Here's how the part is built. I have some questions about the finished solid (model axes, mm). A direction names the side the tool comes from. Give positions to 0.01 mm unless a question says otherwise; leave off trailing zeros. Write each loop counter-clockwise with the first axis right and the second up, starting at its lowest first coordinate (ties: lowest second). Pieces come first, ordered by that corner, then holes. Notation, with made-up numbers: (35.25, 73) -> (76.25, 73) arc R25 cw to (76.25, 102) -> close; hole circle Ø5 at (88.25, -35.5). An arc over 180 degrees is marked (long way). Use one line per item in the form item = value.
```python
from build123d import *

# Parameters (mm, degrees)
SKETCH_W        = 517.525
SKETCH_H        = 563.5625
PAD_DEPTH       = 34.925
SKETCH001_W     = 19.05
SKETCH001_H     = 563.5625
POCKET_DEPTH    = 9.525
POCKET001_DEPTH = 34.926
SKETCH003_W     = 3.175
SKETCH003_H     = 563.5625
PAD001_DEPTH    = 34.925


with BuildPart() as part:
    # Sketch → Pad (new body)
    with BuildSketch(Plane.XY):
        Rectangle(SKETCH_W, SKETCH_H)
    extrude(amount=PAD_DEPTH)

    # Sketch001 (on Face6 of Pad) → Pocket (cut)
    with BuildSketch(Plane.XY.offset(34.925)):
        with Locations((-153.9875, 0)):
            Rectangle(SKETCH001_W, SKETCH001_H)
        with Locations((93.6625, 0)):
            Rectangle(SKETCH001_W, SKETCH001_H)
    extrude(amount=-POCKET_DEPTH, mode=Mode.SUBTRACT)

    # Sketch002 (on Face9 of Pocket) → Pocket001 (cut, through all)
    with BuildSketch(Plane.XY.offset(34.925)):
        with BuildLine():
            ThreePointArc((-7.9375, 161.13125), (-55.5625, 208.75625), (-103.1875, 161.13125))
            Line((-103.1875, 161.13125), (-103.1875, 8.73125))
            ThreePointArc((-103.1875, 8.73125), (-55.5625, -38.89375), (-7.9375, 8.73125))
            Line((-7.9375, 8.73125), (-7.9375, 161.13125))
        make_face()
    extrude(amount=-POCKET001_DEPTH, mode=Mode.SUBTRACT)

    # Sketch003 (on Face9 of Pocket001) → Pad001 (join)
    with BuildSketch(Plane.XY.offset(34.925)):
        with Locations((-34.925, 0)):
            Rectangle(SKETCH003_W, SKETCH003_H)
    extrude(amount=-PAD001_DEPTH)


solid = part.part
```
Q1. I want a section at A-A, the plane y = 20. Write out the boundary of the cut face in (x, z) (1 decimal).
Result set:
outline = (-258.8, 0) -> (-103.2, 0) -> (-103.2, 34.9) -> (-144.5, 34.9) -> (-144.5, 25.4) -> (-163.5, 25.4) -> (-163.5, 34.9) -> (-258.8, 34.9) -> close; (-36.5, 0) -> (-33.3, 0) -> (-33.3, 34.9) -> (-36.5, 34.9) -> close; (-7.9, 0) -> (258.8, 0) -> (258.8, 34.9) -> (103.2, 34.9) -> (103.2, 25.4) -> (84.1, 25.4) -> (84.1, 34.9) -> (-7.9, 34.9) -> close
Q2. I want a section at B-B, the plane z = 15. Count the separate pieces of the cut face and the enclosed holes in it, and give its area (3 significant figures).
Result set:
separate_pieces = 1
enclosed_holes = 2
area = 271,000 mm2
Q3. Will these pins go through, and if not, where does the flat tip stop? pin 1 Ø1 at (x, y) = (3.5, -92.5) entering from -Z; pin 2 Ø5.5 at (x, y) = (96.5, 90.5) entering from +Z.
Result set:
pin_1 = 0
pin_2 = 25.4
Q4. I want a section at D-D, the plane y = -120. Write out the boundary of the cut face in (x, z) (1 decimal), and give its area (3 significant figures).
Result set:
outline = (-258.8, 0) -> (258.8, 0) -> (258.8, 34.9) -> (103.2, 34.9) -> (103.2, 25.4) -> (84.1, 25.4) -> (84.1, 34.9) -> (-144.5, 34.9) -> (-144.5, 25.4) -> (-163.5, 25.4) -> (-163.5, 34.9) -> (-258.8, 34.9) -> close
area = 17,700 mm2
Q5. If I drill on line 1 along X through (y, z) = (139.5, 32); line 2 along X through (y, z) = (251, 32.5); line 3 along X through (y, z) = (74, 10.5), over which ranges is the centre line in solid material (lowest first)? Write a range as from..to.
Result set:
line_1 = -258.76..-163.51, -144.46..-103.19, -36.51..-33.34, -7.94..84.14, 103.19..258.76
line_2 = -258.76..-163.51, -144.46..84.14, 103.19..258.76
line_3 = -258.76..-103.19, -36.51..-33.34, -7.94..258.76
Q6. I want a section at C-C, the plane x = -92.5. Write out the boundary of the cut face in (y, z) (3 decimals), and give its area (3 significant figures).
Result set:
outline = (-281.781, 0) -> (-21.331, 0) -> (-21.331, 34.925) -> (-281.781, 34.925) -> close; (191.194, 0) -> (281.781, 0) -> (281.781, 34.925) -> (191.194, 34.925) -> close
area = 12,300 mm2
Q7. Which directions (+Z, -Z, +X, -X, +Y, -Y) give clear straight access to the entire face, cutting with the end or side of a thin tool? Please do faces 4 (the face through (-154, 4, 25.4)), 5 (the face through (-81.092, 201.335, 17.707)), 6 (the face through (-6, 4, 34.925)).
Result set:
face_4 = +Z, +Y, -Y
face_5 = +Z, -Z
face_6 = +Z, +X, -X, +Y, -Y
Q8. If we mould it in two halves opening along X, with no side actions, what happens to faces 1 (the face through (-258.762, -4, 17)), 2 (the face through (-4, 4, 0)), 3 (the face through (94, 4, 25.4))? For each: +X half, -X half, draft (parallel to the pull), parting line (faces both ways), or undercut.
Result set:
face_1 = -X half
face_2 = draft
face_3 = undercut
